from build123d import *

# Parameters (mm, degrees)
SKETCH_1_W          = 62.3
SKETCH_1_H          = 44.9
EXTRUDE_1_DEPTH     = 33
CUT_EXTRUDE_1_DEPTH = 8
FILLET_1_R          = 3


with BuildPart() as part:
    # Эскиз1 → Бобышка-Вытянуть1 (new body)
    with BuildSketch(Plane(origin=(0, 0, 0), x_dir=(1, 0, 0), z_dir=(0, 1, 0))):
        with Locations((31.15, 22.45)):
            Rectangle(SKETCH_1_W, SKETCH_1_H)
    extrude(amount=EXTRUDE_1_DEPTH)

    # Эскиз3 → Вырез-Вытянуть1 (cut)
    with BuildSketch(Plane(origin=(0, 33, 0), x_dir=(1, 0, 0), z_dir=(0, 1, 0))):
        Polygon((30.3, 18.9), (30.3, 44.9), (0, 44.9), (0, 0), (62.3, 0), (62.3, 18.9), align=None)
    extrude(amount=-CUT_EXTRUDE_1_DEPTH, mode=Mode.SUBTRACT)

    # Скругление1
    fillet_1_edges = [part.edges().sort_by_distance(p)[0] for p in [
        (0, 12.5, -44.9),
        (62.3, 12.5, 0),
        (0, 12.5, 0),
        (30.3, 29, -44.9),
        (30.3, 29, -18.9),
        (62.3, 25, -9.45),
        (62.3, 29, -18.9),
        (31.15, 25, 0),
        (0, 25, -22.45),
        (15.15, 25, -44.9),
        (31.15, 0, -44.9),
        (62.3, 0, -22.45),
        (31.15, 0, 0),
        (0, 0, -22.45),
        (62.3, 16.5, -44.9),
    ]]
    fillet(fillet_1_edges, radius=FILLET_1_R)


solid = part.part
Design review of the part built by this model. Coordinates are the model's own, in mm. A direction names the side the tool comes from. Round coordinates to 2 decimals unless told otherwise and drop trailing zeros. Loops run counter-clockwise (first coordinate to the right, second up) from the corner with the lowest first, then second, coordinate; pieces in that order, holes last. Notation, with made-up numbers: (23, -28) - (71, -28) arc R16 ccw to (71, -4) - close; hole circle Ø11 at (84.25, 57). An arc over 180 degrees is marked (long way). One line per item, written item: value. Start each with the question number.
1) Insertion check: pin 1 Ø6.5 at (y, z) = (28, -31.5) entering from -X; pin 2 Ø12 at (x, z) = (20, -33.5) entering from +Y; pin 3 Ø9 at (x, y) = (44, 27.5) entering from +Z; pin 4 Ø2 at (x, y) = (24, 26.5) entering from -Z. Each pin has a flat end and moves straight along its axis. Give the tip position at first contact, or say it passes through.
2) Consider section D-D on x = 47. Give the boundary of the cut face in (y, z), then the cut area to 3 significant figures.
3) Consider section B-B on z = -13.5. Give the boundary of the cut face in (x, y).
4) For faces 1 (the flat face through (46, 29, -18.9)), 2 (the cylindrical face through (17.94, 24.1, -44.04)), 3 (the cylindrical face through (61.44, 28.65, -19.8)), list the 3-axis set-ups (+Z, -Z, +X, -X, +Y, -Y) from which the entire face can be reached by the end or side of a thin tool; tool diameter is ignored.
5) Consider section C-C on y = 24. Give the boundary of the cut face in (x, z).
6) To check wall thickness, follow L1, parallel to Y at x = 13, z = -25; L2, parallel to X at y = 31, z = -26.5; L3, parallel to Z at x = 42, y = 28. State the ranges of each line that lie inside material, in increasing order. Write a range as from..to.
7) Consider section A-A on x = 15.5. Give the boundary of the cut face in (y, z).
Reported:
1. pin 1: stops at x = 1.8
1. pin 2: stops at y = 25
1. pin 3: stops at z = -0.17
1. pin 4: passes through
2. outline: (0, -41.9) arc R3 ccw to (3, -44.9) - (33, -44.9) - (33, -18.9) - (25, -18.9) - (25, -3) arc R3 ccw to (22, 0) - (3, 0) arc R3 ccw to (0, -3) - close
2. area: 1,320 mm^2
3. outline: (0, 3) arc R3 ccw to (3, 0) - (59.3, 0) arc R3 ccw to (62.3, 3) - (62.3, 22) arc R3 ccw to (59.3, 25) - (3, 25) arc R3 ccw to (0, 22) - close
4. face 1: +Z, +X, -X, +Y
4. face 2: -Z, -X, +Y
4. face 3: +Z, +X, +Y
5. outline: (0.76, -41.9) arc R2.24 ccw to (3, -44.14) - (31.3, -44.14) arc R3 ccw to (33.3, -44.9) - (59.3, -44.9) arc R3 ccw to (62.3, -41.9) - (62.3, -21.9) arc R3 ccw to (61.54, -19.9) - (61.54, -3) arc R2.24 ccw to (59.3, -0.76) - (3, -0.76) arc R2.24 ccw to (0.76, -3) - close
6. L1: y = 0..25
6. L2: x = 30.3..62.3
6. L3: z = -44.9..-18.9
7. outline: (0, -41.9) arc R3 ccw to (3, -44.9) - (22, -44.9) arc R3 ccw to (25, -41.9) - (25, -3) arc R3 ccw to (22, 0) - (3, 0) arc R3 ccw to (0, -3) - close
